Verification items for this drawing (mm, ordinates from the low corner). A direction names the side the tool comes from. Round coordinates to 2 decimals unless told otherwise and drop trailing zeros. Order: outer loops, then holes, each group sorted by start corner. A loop starts at its lowest first (then second) coordinate and runs counter-clockwise, first axis right, second up. Notation, with made-up numbers: (41, -21.5) -> (79, -21.5) arc R19 ccw to (79, 9.5) -> close; hole circle Ø11 at (65, 53). An arc over 180 degrees is marked (long way). Put each result on its own line as item: value.
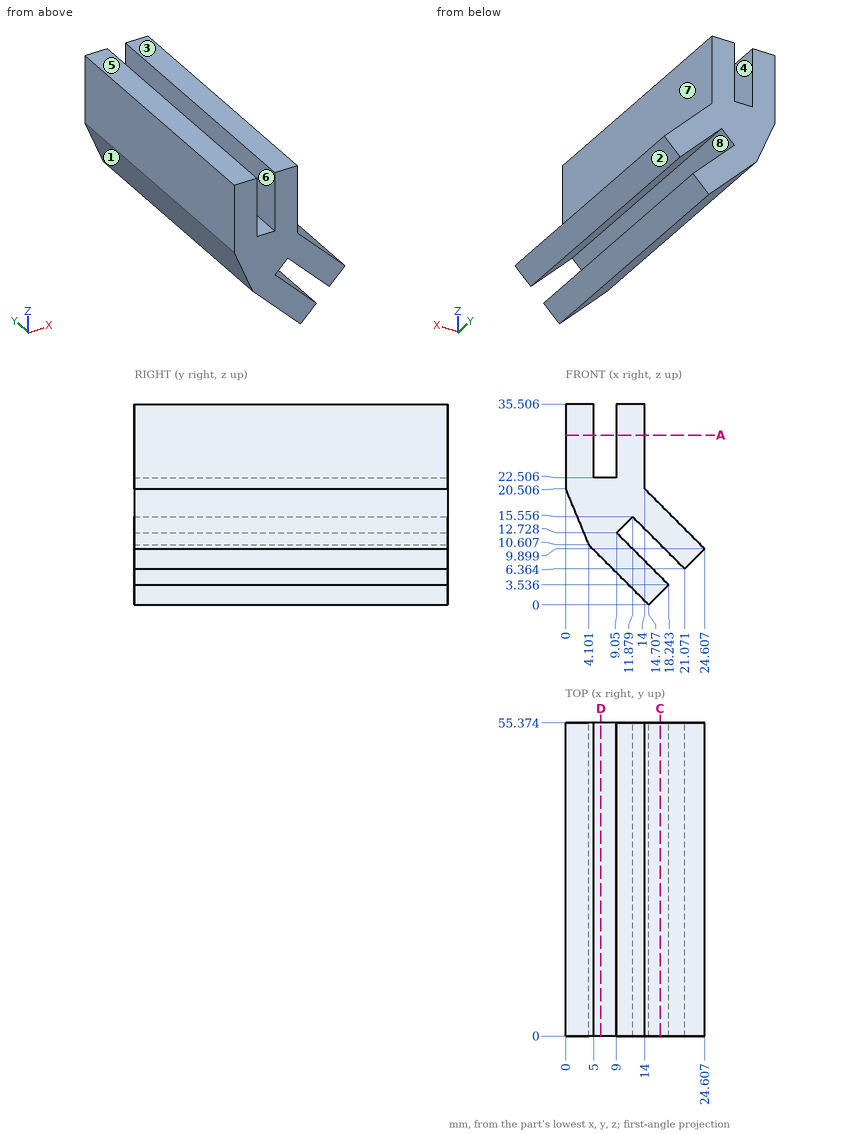
Item 1: Section check C-C on x = 16.75. Record the boundary of the cut face in (y, z) (1 decimal), then the cut area to 3 significant figures.
Check sheet entries:
outline: (0, 2) -> (55.4, 2) -> (55.4, 5) -> (0, 5) -> close; (0, 10.7) -> (55.4, 10.7) -> (55.4, 17.8) -> (0, 17.8) -> close
area: 557 mm^2
Item 2: Section check A-A on z = 30. Record the boundary of the cut face in (x, y) (1 decimal), then the cut area to 3 significant figures.
Check sheet entries:
outline: (0, 0) -> (5, 0) -> (5, 55.4) -> (0, 55.4) -> close; (9, 0) -> (14, 0) -> (14, 55.4) -> (9, 55.4) -> close
area: 554 mm^2
Item 3: Material ranges on L1, parallel to X at y = 46, z = 27; L2, parallel to Z at x = 15.25, y = 10.5 (1 decimal); L3, parallel to X at y = 3, z = 22, recorded low to high. Write a range as [from, to].
Check sheet entries:
L1: x = [0, 5], [9, 14]
L2: z = [0.5, 6.5], [12.2, 19.3]
L3: x = [0, 14]
Item 4: Release check for a two-part mould opening along X. For the marked faces 1, 2, 3 and 4 record: +X half, -X half, draft (parallel to the pull), parting line (faces both ways), or undercut.
Check sheet entries:
face 1: -X half
face 2: +X half
face 3: draft
face 4: undercut
Item 5: Gauge pin test, flat ends, axial feed: pin 1 Ø1 at (y, z) = (7.5, 11) entering from -X; pin 2 Ø10.5 at (y, z) = (29, 27) entering from +X; pin 3 Ø6 at (x, y) = (21, 26.5) entering from +Z (1 decimal). Record the tip position at first contact, or that the pin passes through.
Check sheet entries:
pin 1: stops at x = 3.73
pin 2: stops at x = 14
pin 3: stops at z = 16.5
Item 6: Section check D-D on x = 6.25. Record the boundary of the cut face in (y, z) (1 decimal).
Check sheet entries:
outline: (0, 8.5) -> (55.4, 8.5) -> (55.4, 22.5) -> (0, 22.5) -> close
Item 7: Tool access check on the marked faces 5, 6, 7 and 8. Record the directions out of +Z, -Z, +X, -X, +Y, -Y that give a thin tool (end or side, any length) a straight path to the whole face; none if there is none.
Check sheet entries:
face 5: +Z, +X, -X, +Y, -Y
face 6: +Z, +Y, -Y
face 7: +Z, +X, +Y, -Y
face 8: +Y, -Y
